Build history of the part. All positions in model axes, mm. A direction names the side the tool comes from. Coordinates: 2 decimals unless noted, no trailing zeros. Order: outer loops, then holes, each group sorted by start corner. A loop starts at its lowest first (then second) coordinate and runs counter-clockwise, first axis right, second up. Notation, with made-up numbers: (82.25, -2.75) -> (123.25, -2.75) arc R8 ccw to (123.25, 11.25) -> close; hole circle Ø9 at (-23, 15.25). An arc over 180 degrees is marked (long way). Write each question's results on one line, items separated by ' | '.
Autodesk Inventor part; units mm, degrees
ref_plane "Work Plane10" through (-7.1266, 5.8946, 10.4647) normal (0.9341198, -0.2351055, -0.2685995) x (-0.2685995, 0.0326501, -0.9626984)
ref_plane "Work Plane12" through (-19.3217, -20.3191, 0.3055) normal (-0.2351055, -0.9714213, 0.0326501) x (0.9341198, -0.2351055, -0.2685995)
ref_plane "YZ Plane" through (0, 0, 0) normal (1, 0, 0) x (0, 1, 0)
ref_plane "Work Plane10" through (-7.1266, 5.8946, 10.4647) normal (0.9341198, -0.2351055, -0.2685995) x (-0.2685995, 0.0326501, -0.9626984)
sketch "Sketch2" plane through (-7.1266, 5.8946, 10.4647) normal (0.9341198, -0.2351055, -0.2685995) x (-0.2685995, 0.0326501, -0.9626984)
  line L0 (0, 5) -> (12.2, 5)
  line L1 (12.2, 5) -> (12.2, 0)
  line L2 (12.2, 0) -> (0, 0)
  line L3 (0, 0) -> (0, 5)
  line L4 (12.2, -28) -> (0, -28)
  line L5 (0, -28) -> (0, -23)
  line L6 (0, -23) -> (12.2, -23)
  line L7 (12.2, -23) -> (12.2, -28)
  point P0 (7.9677, -3.709)
extrude "Extrusion2" add sketch "Sketch2" along normal blind 20
ref_plane "Work Plane12" through (-19.3217, -20.3191, 0.3055) normal (-0.2351055, -0.9714213, 0.0326501) x (0.9341198, -0.2351055, -0.2685995)
sketch "Sketch4" plane through (-19.3217, -20.3191, 0.3055) normal (-0.2351055, -0.9714213, 0.0326501) x (0.9341198, -0.2351055, -0.2685995)
  line L0 (7.7802, 8.6462) -> (19.9601, 8.6462)
  line L1 (19.9601, 8.6462) -> (19.9601, 3.5538)
  line L2 (19.9601, 3.5538) -> (7.7802, 3.5538)
  line L3 (7.7802, 3.5538) -> (7.7802, 8.6462)
  line L4 (43.7973, 6.1) -> (-30.4435, 6.1)
  point P0 (13.3537, 4.2323)
  point P1 (7.7802, 6.1)
extrude "Extrusion4" cut sketch "Sketch4" against normal up to surface (5 mm away)
ref_plane "Work Plane11" through (11.5558, 1.1925, 5.0927) normal (0.9341198, -0.2351055, -0.2685995) x (-0.2685995, 0.0326501, -0.9626984)
sketch "Sketch5" plane through (11.5558, 1.1925, 5.0927) normal (0.9341198, -0.2351055, -0.2685995) x (-0.2685995, 0.0326501, -0.9626984)
  line L0 (12.2, 5) -> (0, 5)
  line L1 (0, 5) -> (0, -28)
  line L2 (0, -28) -> (12.2, -28)
  line L3 (12.2, -28) -> (12.2, 5)
  point P0 (7.9677, -3.709)
extrude "Extrusion5" add sketch "Sketch5" along normal blind 4.25
hole "Hole1" at (-14.7602, -18.6775, 5.4248) direction (0.9341198, -0.2351055, -0.2685995) diameter 2 depth 8 tip angle 118
hole "Hole3" at (-8.1773, 8.5223, 4.5106) direction (0.9341198, -0.2351055, -0.2685995) diameter 2 depth 8 tip angle 118
thread "Thread1"
thread "Thread2"
hole "Hole4" at (7.8922, -24.3788, -1.0887) direction (-0.9341198, 0.2351055, 0.2685995) diameter 2 depth 8 tip angle 118
hole "Hole5" at (14.4752, 2.821, -2.0029) direction (-0.9341198, 0.2351055, 0.2685995) diameter 2 depth 8 tip angle 118
thread "Thread3"
properties part number "servo_attachement"
Item 1: Slice it at A-A, the plane z = 8. List the corners of the cut face in (x, y) (3 decimals).
Answer:
outline: (-14.652, -21.191) -> (-1.959, -24.263) -> (-1.351, -19.263) -> (-13.431, -16.339) -> close; (-7.814, 5.978) -> (1.445, 3.737) -> (2.053, 8.737) -> (-6.593, 10.83) -> close
Item 2: Pin check, flat tips, straight feed: pin 1 (5 mm diameter, centred on x = 4, z = -4, fed in from +Y); pin 2 (10 mm diameter, centred on y = -3.5, z = 8.5, fed in from -X); pin 3 (6 mm diameter, centred on x = 10.5, z = 6, fed in from +Y). Stop position of each tip, or through.
Answer:
pin 1: stops at y = 8.47 | pin 2: stops at x = 9.44 | pin 3: stops at y = 7.36
Item 3: Pull direction X, two halves, no side cores. Call faces 1 (the conical face through (6.504, 4.869, 0.117)), 2 (the conical face through (-0.2, 6.5, 2.4)), 3 (the flat face through (11.26, -10.56, -1.47)), 4 (the flat face through (-7.78, 8.51, 5.9)): released by +X, released by -X, zero draft, split by the parting line, or undercut.
Answer:
face 1: undercut | face 2: undercut | face 3: released by +X | face 4: released by -X
Item 4: Drill centre lines: line 1 (Y direction, x = -0.5, z = -2.25); line 2 (X direction, y = -20, z = 3); line 3 (Z direction, x = -8, y = -18.5). Where is each one in solid material? Low to high. Write a range as from..to.
Answer:
line 1: y = -24.96..-19.81, 3.86..9.01 | line 2: x = -15.79..-10.14, 5.62..10.17 | line 3: z = -2.79..0.9, 6.19..9.88
Item 5: Slice it at D-D, the plane y = -13.5. List the corners of the cut face in (x, z) (3 decimals).
Answer:
outline: (4.627, -6.145) -> (8.838, -7.32) -> (12.212, 4.411) -> (8, 5.587) -> close
Item 6: Slice it at C-C, the plane z = -3.5. List the corners of the cut face in (x, y).
Answer:
outline: (-6.09, -23.65) -> (6.61, -26.72) -> (14.67, 5.3) -> (-2.08, 9.35) -> (-2.68, 4.35) -> (9.16, 1.48) -> (3.54, -20.83) -> (-5.48, -18.65) -> close
Item 7: Slice it at B-B, the plane x = -5. State how many separate pieces and enclosed holes the cut face has, and give its area (4 significant figures).
Answer:
separate pieces: 3 | enclosed holes: 1 | area: 100.0 mm^2
Item 8: Tool access for faces 5 (the flat face through (-14.365, -18.691, 6.811)), 6 (the flat face through (1.855, -22.855, 1.86)): list every direction of +Z, -Z, +X, -X, +Y, -Y with a clear straight run to the whole face (end or side of a thin tool).
Answer:
face 5: +Z, -X, +Y | face 6: none
